from build123d import *

# Parameters (mm, degrees)
SKICA1_R                      = 12.3
P_IDAT_VYSUNUT_M1_DEPTH       = 1.5
ODEBRAT_START                 = 1.5
SKICA1_6_R                    = 1.75
ODEBRAT_VYSUNUT_M3_DEPTH      = 0.8
P_IDAT_VYSUNUT_M3_DEPTH       = 3
P_IDAT_START                  = 1
P_IDAT_VYSUNUT_M4_DEPTH       = 2
ZKOSEN_1_SIZE                 = 0.4
KRUHOV_POLE1_COUNT            = 2
ZKOSEN_1_OF_KRUHOV_POLE1_SIZE = 0.4
ODEBRAT_VYSUNUT_M2_DEPTH      = 0.5
ODEBRAT_VYSUNUT_M1_DEPTH      = 1.2
ODEBRAT_VYSUNUT_M1_DEPTH_BACK = 1.2


with BuildPart() as part:
    # Skica1 → P_idat vysunut_m1 (new body)
    with BuildSketch(Plane.XY):
        Circle(SKICA1_R)
    extrude(amount=P_IDAT_VYSUNUT_M1_DEPTH)

    # Skica1_6 → Odebrat vysunut_m3 (cut)
    with BuildSketch(Plane.XY.offset(ODEBRAT_START)):
        with Locations((-9.85, 0)):
            Circle(SKICA1_6_R)
        with Locations((9.85, 0)):
            Circle(SKICA1_6_R)
    extrude(amount=-ODEBRAT_VYSUNUT_M3_DEPTH, mode=Mode.SUBTRACT)

    # Skica1_5 → P_idat vysunut_m3 (add)
    with BuildSketch(Plane.XY):
        with BuildLine():
            Line((-2, 10.867497412), (-1.837104072, 9.982361876))
            ThreePointArc((-1.837104072, 9.982361876), (0, 10.15), (1.837104072, 9.982361876))
            Line((1.837104072, 9.982361876), (2, 10.867497412))
            ThreePointArc((2, 10.867497412), (0, 11.05), (-2, 10.867497412))
        make_face()
    p_idat_vysunut_m3 = extrude(amount=-P_IDAT_VYSUNUT_M3_DEPTH)

    # Skica2 → P_idat vysunut_m4 (add)
    with BuildSketch(Plane(origin=(0, 0, 0), x_dir=(-1, 0, 0), z_dir=(0, 0, -1)).offset(P_IDAT_START)):
        with BuildLine():
            Line((-2, 10.867497412), (-2.199095023, 11.949329734))
            ThreePointArc((-2.199095023, 11.949329734), (0, 12.15), (2.199095023, 11.949329734))
            Line((2.199095023, 11.949329734), (2, 10.867497412))
            ThreePointArc((2, 10.867497412), (0, 11.05), (-2, 10.867497412))
        make_face()
    p_idat_vysunut_m4 = extrude(amount=P_IDAT_VYSUNUT_M4_DEPTH)

    # Zkosen_1
    zkosen_1_edges = [part.edges().sort_by_distance(p)[0] for p in [
        (0, 10.15, -3),
    ]]
    chamfer(zkosen_1_edges, length=ZKOSEN_1_SIZE)

    # Kruhov_ pole1: P_idat vysunut_m3, P_idat vysunut_m4 ×2 about axis
    kruhov_pole1_axis = Axis((0, 0, 0), (0, 0, 1))
    for i in range(1, KRUHOV_POLE1_COUNT):
        add(p_idat_vysunut_m3.rotate(kruhov_pole1_axis, i * 360 / KRUHOV_POLE1_COUNT))
        add(p_idat_vysunut_m4.rotate(kruhov_pole1_axis, i * 360 / KRUHOV_POLE1_COUNT))

    # Zkosen_1 of Kruhov_ pole1
    zkosen_1_of_kruhov_pole1_edges = [part.edges().sort_by_distance(p)[0] for p in [
        (0, -10.15, -3),
    ]]
    chamfer(zkosen_1_of_kruhov_pole1_edges, length=ZKOSEN_1_OF_KRUHOV_POLE1_SIZE)

    # Skica3 → Odebrat vysunut_m2 (cut)
    with BuildSketch(Plane.XY.offset(1.5)):
        with BuildLine():
            Line((-3.166666667, 8.956685895), (-3, 8.485281374))
            ThreePointArc((-3, 8.485281374), (0, 9), (3, 8.485281374))
            Line((3, 8.485281374), (2.883333333, 8.15529821))
            Line((2.883333333, 8.15529821), (5.144077535, 7.992400535))
            Line((5.144077535, 7.992400535), (3.283333333, 9.28666906))
            Line((3.283333333, 9.28666906), (3.166666667, 8.956685895))
            ThreePointArc((3.166666667, 8.956685895), (0, 9.5), (-3.166666667, 8.956685895))
        make_face()
    extrude(amount=-ODEBRAT_VYSUNUT_M2_DEPTH, mode=Mode.SUBTRACT)

    # Skica4 → Odebrat vysunut_m1 (cut, two sides)
    with BuildSketch(Plane(origin=(0, 0, 0), x_dir=(0, 0, -1), z_dir=(1, 0, 0))) as odebrat_vysunut_m1_sk:
        with BuildLine():
            Line((-1.5, 5), (-1.5, -5))
            ThreePointArc((-1.5, -5), (-0.642135624, 0), (-1.5, 5))
        make_face()
    extrude(amount=ODEBRAT_VYSUNUT_M1_DEPTH, mode=Mode.SUBTRACT)
    extrude(odebrat_vysunut_m1_sk.sketch, amount=-ODEBRAT_VYSUNUT_M1_DEPTH_BACK, mode=Mode.SUBTRACT)


solid = part.part
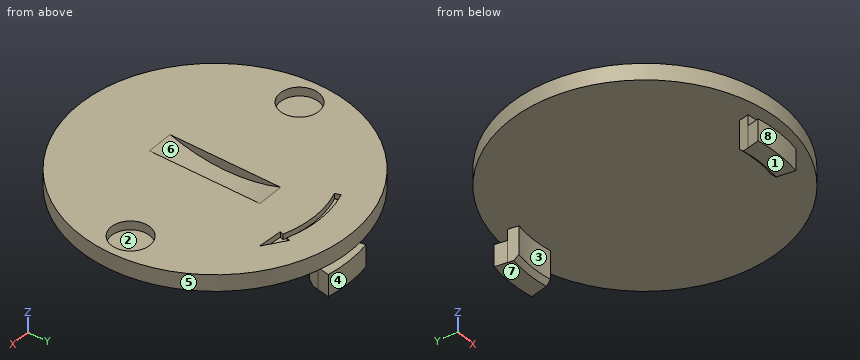
Input: part model. Units: mm. Frame: model coordinates. Face numbers are marked on the shaded views. A direction names the side the tool comes from. Coordinates: 2 decimals unless noted, no trailing zeros. Loops run counter-clockwise (first coordinate to the right, second up) from the corner with the lowest first, then second, coordinate; pieces in that order, holes last.
Q1. Contact query for flat-ended pins moving along their axis: pin 1 (3 mm diameter, centred on x = 10, y = -1, fed in from +Z); pin 2 (0.7 mm diameter, centred on y = -1, z = 1, fed in from +X); pin 3 (0.7 mm diameter, centred on y = -1.5, z = 1, fed in from -X); pin 4 (4.5 mm diameter, centred on x = 9.85, y = 0, fed in from -Z). Output: stop coordinate, or through.
Q2. Set-up query: the marked faces 1, 2, 3, 4 and 5. Return all of +Z, -Z, +X, -X, +Y, -Y with unobstructed straight access to the full face (end or side cutting, diameter ignored); none if empty.
Q3. Cut plane D-D (z = -0.5). Output: boundary loops of the cut face in (x, y), then the cut area to 3 significant figures.
Q4. Material intervals for line 1 (Y direction, x = 10, z = 1.05); line 2 (Y direction, x = 9.85, z = 0.95); line 3 (Z direction, x = 4.25, y = -4.5), sorted ascending.
Q5. Cut plane A-A (z = -2.2). Output: boundary loops of the cut face in (x, y).
Q6. Cut plane C-C (x = 0). Output: boundary loops of the cut face in (y, z), then the cut area to 3 significant figures.
Q7. Cut plane B-B (y = 0). Output: boundary loops of the cut face in (x, z).
Q8. Draft query along X for the marked faces 6, 7 and 8. Return one class per face: +X half, -X half, draft (parallel to the pull), parting line (faces both ways), or undercut.
Working result:
1. pin 1: stops at z = 1.5
1. pin 2: stops at x = 12.28
1. pin 3: stops at x = -12.25
1. pin 4: stops at z = 0
2. face 1: -Z, +X, -X, +Y, -Y
2. face 2: +Z
2. face 3: -Z
2. face 4: -Z, +Y
2. face 5: +Z, -Z
3. outline: (-2, -10.87) arc R11.05 ccw to (2, -10.87) - (1.84, -9.98) arc R10.15 cw to (-1.84, -9.98) - close; (-2, 10.87) - (-1.84, 9.98) arc R10.15 cw to (1.84, 9.98) - (2, 10.87) arc R11.05 ccw to start
3. area: 6.95 mm2
4. line 1: y = -7.16 to -1.74, 1.74 to 7.16
4. line 2: y = -7.37 to -1.75, 1.75 to 7.37
4. line 3: z = 0 to 1.5
5. outline: (-2.2, -11.95) arc R12.15 ccw to (2.2, -11.95) - (1.84, -9.98) arc R10.15 cw to (-1.84, -9.98) - close; (-2.2, 11.95) - (-1.84, 9.98) arc R10.15 cw to (1.84, 9.98) - (2.2, 11.95) arc R12.15 ccw to start
6. outline: (-12.3, 0) - (-11.05, 0) - (-11.05, -1) - (-12.15, -1) - (-12.15, -3) - (-10.55, -3) - (-10.15, -2.6) - (-10.15, 0) - (10.15, 0) - (10.15, -2.6) - (10.55, -3) - (12.15, -3) - (12.15, -1) - (11.05, -1) - (11.05, 0) - (12.3, 0) - (12.3, 1.5) - (9.5, 1.5) - (9.5, 1) - (9, 1) - (9, 1.5) - (5, 1.5) arc R15 cw to (-5, 1.5) - (-12.3, 1.5) - close
6. area: 40.5 mm2
7. outline: (-12.3, 0) - (12.3, 0) - (12.3, 1.5) - (11.6, 1.5) - (11.6, 0.7) - (8.1, 0.7) - (8.1, 1.5) - (1.2, 1.5) - (1.2, 0.64) - (-1.2, 0.64) - (-1.2, 1.5) - (-8.1, 1.5) - (-8.1, 0.7) - (-11.6, 0.7) - (-11.6, 1.5) - (-12.3, 1.5) - close
8. face 6: undercut
8. face 7: draft
8. face 8: parting line
